```python
from build123d import *

# Parameters (mm, degrees)
EXTRUDE_1_DEPTH        = 150
SHELL_START            = 2
SHELL_1_DEPTH          = 146
SKETCH_3_W             = 500
SKETCH_3_H             = 2
EXTRUDE_2_DEPTH        = 10
CUT_EXTRUDE_1_DEPTH    = 10
SKETCH_5_R             = 2.5
CUT_EXTRUDE_2_DEPTH    = 2
PATTERN_LINEAR_1_COUNT = 5
PATTERN_LINEAR_1_PITCH = 70
SKETCH_6_R             = 2
CUT_EXTRUDE_3_DEPTH    = 2
SKETCH_7_R             = 4
CUT_EXTRUDE_4_DEPTH    = 2
CUT_EXTRUDE_5_REACH    = 297
SKETCH_8_R             = 4
SKETCH_9_W             = 28.6
SKETCH_9_H             = 48
SKETCH_9_W_2           = 18.2
SKETCH_9_H_2           = 37.6
EXTRUDE_3_DEPTH        = 4
CHAMFER_1_SIZE         = 4
SKETCH_11_W            = 34.8
SKETCH_11_H            = 29.2
SKETCH_11_W_2          = 30.8
SKETCH_11_H_2          = 25.2
EXTRUDE_4_DEPTH        = 3
CUT_EXTRUDE_6_REACH    = 304.324
SKETCH_11_2_W          = 30.8
SKETCH_11_2_H          = 25.2
EXTRUDE_5_REACH        = 274.555
SKETCH_14_R            = 1.5
SKETCH_9_2_W           = 18.2
SKETCH_9_2_H           = 37.6
EXTRUDE_6_DEPTH        = 3


# Read off the part's stored shape, not the designer's step: 抽壳1
with BuildPart() as part:
    # 草图1 → 凸台-拉伸1 (new body)
    with BuildSketch(Plane.XY):
        Polygon((-250, 5), (-230, 35), (-130, 35), (-130, 33), (150, 33), (150, 35), (250, 35), (250, -35), (-250, -35), align=None)
    extrude(amount=EXTRUDE_1_DEPTH)

    # 抽壳1 outline → 抽壳1 (cut)
    with BuildSketch(Plane.XY.offset(SHELL_START)):
        Polygon((248, 33), (-228.929632483, 33), (-248, 4.394448725), (-248, -33), (248, -33), align=None)
    extrude(amount=SHELL_1_DEPTH, mode=Mode.SUBTRACT)

    # 草图3 → 凸台-拉伸2 (add)
    with BuildSketch(Plane.XZ.offset(35)):
        with Locations((0, 149)):
            Rectangle(SKETCH_3_W, SKETCH_3_H)
    extrude_2 = extrude(amount=EXTRUDE_2_DEPTH)

    # 草图4 → 切除-拉伸1 (cut)
    with BuildSketch(Plane.XY.offset(150)):
        Polygon((-150, -45), (-170, -35), (-250, -35), (-250, -45), align=None)
        Polygon((250, -35), (200, -35), (180, -45), (250, -45), align=None)
    cut_extrude_1 = extrude(amount=-CUT_EXTRUDE_1_DEPTH, mode=Mode.SUBTRACT)

    # 镜向1: 凸台-拉伸2, 切除-拉伸1 across plane
    add(extrude_2.mirror(Plane(origin=(0, 0, 75), x_dir=(1, 0, 0), z_dir=(0, 0, -1))))
    add(cut_extrude_1.mirror(Plane(origin=(0, 0, 75), x_dir=(1, 0, 0), z_dir=(0, 0, -1))), mode=Mode.SUBTRACT)

    # 草图5 → 切除-拉伸2 (cut)
    with BuildSketch(Plane.XY.offset(150)):
        with Locations((-135, -39)):
            Circle(SKETCH_5_R)
    cut_extrude_2 = extrude(amount=-CUT_EXTRUDE_2_DEPTH, mode=Mode.SUBTRACT)

    # 阵列(线性)1: 切除-拉伸2 ×5
    with Locations(*[(i * PATTERN_LINEAR_1_PITCH, 0, 0) for i in range(1, PATTERN_LINEAR_1_COUNT)]):
        add(cut_extrude_2, mode=Mode.SUBTRACT)

    # 草图6 → 切除-拉伸3 (cut)
    with BuildSketch(Plane.XY.offset(150)):
        with Locations((-135, 5)):
            Circle(SKETCH_6_R)
        with Locations((25, 5)):
            Circle(SKETCH_6_R)
        with Locations((155, 5)):
            Circle(SKETCH_6_R)
    extrude(amount=-CUT_EXTRUDE_3_DEPTH, mode=Mode.SUBTRACT)

    # 草图7 → 切除-拉伸4 (cut)
    with BuildSketch(Plane.XY.offset(150)):
        with Locations((-90, 5)):
            Circle(SKETCH_7_R)
        with Locations((90, 5)):
            Circle(SKETCH_7_R)
    extrude(amount=-CUT_EXTRUDE_4_DEPTH, mode=Mode.SUBTRACT)

    # 草图8 → 切除-拉伸5 (cut, up to next)
    with BuildSketch(Plane.XY.offset(150), mode=Mode.PRIVATE) as cut_extrude_5_sk1:
        with Locations((-210, 0)):
            Circle(SKETCH_8_R)
    cut_extrude_5_tool1 = extrude(cut_extrude_5_sk1.sketch, amount=-CUT_EXTRUDE_5_REACH, mode=Mode.PRIVATE) & part.part
    add(cut_extrude_5_tool1.solids().sort_by_distance((-210, 0, 150))[0], mode=Mode.SUBTRACT)

    # 草图9 → 凸台-拉伸3 (add)
    with BuildSketch(Plane(origin=(0, 35, 0), x_dir=(1, 0, 0), z_dir=(0, 1, 0))):
        with Locations((-188.276603419, -99.2)):
            Rectangle(SKETCH_9_W, SKETCH_9_H)
        with Locations((-188.276603419, -99.2)):
            Rectangle(SKETCH_9_W_2, SKETCH_9_H_2, mode=Mode.SUBTRACT)
    extrude(amount=EXTRUDE_3_DEPTH)

    # 倒角1
    chamfer_1_edges = [part.edges().sort_by_distance(p)[0] for p in [
        (-188.276603419, 39, 80.4),
        (-179.176603419, 39, 99.2),
        (-188.276603419, 39, 118),
        (-197.376603419, 39, 99.2),
    ]]
    chamfer(chamfer_1_edges, length=CHAMFER_1_SIZE - 0.0001)  # a hair under: the kernel refuses the full size

    # 草图11 → 凸台-拉伸4 (add)
    with BuildSketch(Plane(origin=(0, 35, 0), x_dir=(1, 0, 0), z_dir=(0, 1, 0))):
        with Locations((-188.276603419, -38.6)):
            Rectangle(SKETCH_11_W, SKETCH_11_H)
        with Locations((-188.276603419, -38.6)):
            Rectangle(SKETCH_11_W_2, SKETCH_11_H_2, mode=Mode.SUBTRACT)
    extrude(amount=EXTRUDE_4_DEPTH)

    # 草图11<2> → 切除-拉伸6 (cut, up to next)
    with BuildSketch(Plane(origin=(0, 35, 0), x_dir=(1, 0, 0), z_dir=(0, 1, 0)), mode=Mode.PRIVATE) as cut_extrude_6_sk1:
        with Locations((-188.276603419, -38.6)):
            Rectangle(SKETCH_11_2_W, SKETCH_11_2_H)
    cut_extrude_6_tool1 = extrude(cut_extrude_6_sk1.sketch, amount=-CUT_EXTRUDE_6_REACH, mode=Mode.PRIVATE) & part.part
    add(cut_extrude_6_tool1.solids().sort_by_distance((-188.276603, 35, 38.6))[0], mode=Mode.SUBTRACT)

    # 草图14 → 凸台-拉伸5 (add, up to next)
    with BuildSketch(Plane(origin=(0, 0, 51.2), x_dir=(-1, 0, 0), z_dir=(0, 0, -1)), mode=Mode.PRIVATE) as extrude_5_sk1:
        with Locations(Location((188.276603419, 35.5, 0), (0, 0, 180))):
            Circle(SKETCH_14_R)
    extrude_5_tool1 = extrude(extrude_5_sk1.sketch, amount=EXTRUDE_5_REACH, mode=Mode.PRIVATE) - part.part
    add(extrude_5_tool1.solids().sort_by_distance((-188.276603, 35.5, 51.2))[0])

    # 草图9<2> → 凸台-拉伸6 (add)
    with BuildSketch(Plane(origin=(0, 35, 0), x_dir=(1, 0, 0), z_dir=(0, 1, 0))):
        with Locations((-188.276603419, -99.2)):
            Rectangle(SKETCH_9_2_W, SKETCH_9_2_H)
    extrude(amount=-EXTRUDE_6_DEPTH)


solid = part.part
```
Read the model definition and answer for the solid it produces. Units are mm, in the model's axes. A direction names the side the tool comes from. Give positions to 0.01 mm unless a question says otherwise; leave off trailing zeros. Loops run counter-clockwise (first coordinate to the right, second up) from the corner with the lowest first, then second, coordinate; pieces in that order, holes last.
Item 1: The part is cut by section A-A (y = -15). Write down the section's boundary in (x, z), and give its area (3 significant figures).
Item 2: Each of these flat-tipped pins is pushed along its axis until it touches: pin 1 Ø3 at (x, z) = (163, 41.5) entering from +Y; pin 2 Ø3 at (x, z) = (-113, 74) entering from +Y; pin 3 Ø1.2 at (x, y) = (-191, 36.5) entering from -Z. Where does it stop, or does it pass through?
Item 3: The mould has two halves that part along Z. Classify faces 1 (the flat face through (-188, 32, 99)), 2 (the flat face through (199, 35, 74)), 3 (the flat face through (-3, -4, 150)): released by +Z, released by -Z, zero draft, split by the parting line, or undercut.
Item 4: The part is cut by section D-D (x = 15). Write down the section's boundary in (y, z), and give its area (3 significant figures).
Item 5: The part is cut by section C-C (z = 94.5). Write down the section's boundary in (x, y), and give its area (3 significant figures).
Item 6: Find the intervals of material crossed by line 1 along Y through (x, z) = (-135, 149.1); line 2 along Z through (x, y) = (205.5, -19); line 3 along Y through (x, z) = (90, 149), in increasing order.
Item 7: The part is cut by section B-B (z = 40.5). Write down the section's boundary in (x, y), and give its area (3 significant figures).
Item 8: For faces 4 (the flat face through (-188, 35, 99)), 5 (the cylindrical face through (-94, 5, 149)), 6 (the flat face through (-3, -33, 74)), 7 (the flat face through (-192, 38, 52)), determine the directions among +Z, -Z, +X, -X, +Y, -Y from which every point of the face is accessible in a straight line to the end or side of a thin tool.
Taken from the geometry:
1. outline: (-250, 0) - (250, 0) - (250, 150) - (-250, 150) - close; hole (-248, 2) - (248, 2) - (248, 148) - (-248, 148) - close
1. area: 2,580 mm2
2. pin 1: stops at y = 35
2. pin 2: stops at y = -33
2. pin 3: stops at z = 24
3. face 1: undercut
3. face 2: zero draft
3. face 3: released by +Z
4. outline: (-45, 0) - (33, 0) - (33, 2) - (-33, 2) - (-33, 148) - (33, 148) - (33, 150) - (-45, 150) - (-45, 148) - (-35, 148) - (-35, 2) - (-45, 2) - close
4. area: 604 mm2
5. outline: (-250, -35) - (250, -35) - (250, 35) - (150, 35) - (150, 33) - (248, 33) - (248, -33) - (-248, -33) - (-248, 4.39) - (-228.93, 33) - (-197.38, 33) - (-197.38, 32) - (-179.18, 32) - (-179.18, 33) - (-130, 33) - (-130, 35) - (-173.98, 35) - (-173.98, 39) - (-175.18, 39) - (-179.18, 35) - (-197.38, 35) - (-201.38, 39) - (-202.58, 39) - (-202.58, 35) - (-230, 35) - (-250, 5) - close
5. area: 1,720 mm2
6. line 1: y = -45 to -41.5, -36.5 to 3, 7 to 35
6. line 2: z = 0 to 2, 148 to 150
6. line 3: y = -45 to 1, 9 to 33
7. outline: (-250, -35) - (250, -35) - (250, 35) - (150, 35) - (150, 33) - (248, 33) - (248, -33) - (-248, -33) - (-248, 4.39) - (-228.93, 33) - (-203.68, 33) - (-203.68, 38) - (-205.68, 38) - (-205.68, 35) - (-230, 35) - (-250, 5) - close; circle Ø3 at (-188.28, 35.5); (-172.88, 33) - (-130, 33) - (-130, 35) - (-170.88, 35) - (-170.88, 38) - (-172.88, 38) - close
7. area: 1,630 mm2
8. face 4: +Y
8. face 5: +Z
8. face 6: none
8. face 7: -Z, +X, -X, +Y
